Source: CAD feature listing. Evaluate the final solid. Frame: model axes, mm. A direction names the side the tool comes from. Round coordinates to 2 decimals unless told otherwise and drop trailing zeros. Loops run counter-clockwise (first coordinate to the right, second up) from the corner with the lowest first, then second, coordinate; pieces in that order, holes last. Notation, with made-up numbers: M -38.75,-36 L -33.75,-36 A3 cw -33.75,-32 Z; hole C 65.5,-8.75 d5. An arc over 180 degrees is marked long. Answer as a JSON object with one key per item and string values.
from build123d import *

# Parameters (mm, degrees)
SKETCH_1_R          = 30
SKETCH_1_R_2        = 1.5
SKETCH_1_R_3        = 3.5
EXTRUDE_1_DEPTH     = 20
SKETCH_2_R          = 21
CUT_EXTRUDE_1_DEPTH = 17
CUT_EXTRUDE_START   = -0.1
SKETCH_3_R          = 30
SKETCH_3_R_2        = 22.5
CUT_EXTRUDE_2_DEPTH = 0.1
FILLET_1_R          = 0.5


with BuildPart() as part:
    # 草图1 → 凸台-拉伸1 (new body)
    with BuildSketch(Plane(origin=(0, 0, 0), x_dir=(1, 0, 0), z_dir=(0, 1, 0))):
        with Locations(Location((0, 0, 0), (0, 0, 270))):
            Circle(SKETCH_1_R)
        with Locations(Location((0, 6, 0), (0, 0, 270))):
            Circle(SKETCH_1_R_2, mode=Mode.SUBTRACT)
        with Locations(Location((0, 0, 0), (0, 0, 270))):
            Circle(SKETCH_1_R_3, mode=Mode.SUBTRACT)
        with Locations(Location((6, 0, 0), (0, 0, 270))):
            Circle(SKETCH_1_R_2, mode=Mode.SUBTRACT)
        with Locations(Location((0, -6, 0), (0, 0, 270))):
            Circle(SKETCH_1_R_2, mode=Mode.SUBTRACT)
        with Locations(Location((-6, 0, 0), (0, 0, 270))):
            Circle(SKETCH_1_R_2, mode=Mode.SUBTRACT)
    extrude(amount=EXTRUDE_1_DEPTH)

    # 草图2 → 切除-拉伸1 (cut)
    with BuildSketch(Plane(origin=(0, 0, 0), x_dir=(-1, 0, 0), z_dir=(0, -1, 0))):
        with Locations(Location((0, 0, 0), (0, 0, 90))):
            Circle(SKETCH_2_R)
    extrude(amount=-CUT_EXTRUDE_1_DEPTH, mode=Mode.SUBTRACT)

    # 草图3 → 切除-拉伸2 (cut)
    with BuildSketch(Plane(origin=(0, 20, 0), x_dir=(1, 0, 0), z_dir=(0, 1, 0)).offset(CUT_EXTRUDE_START)):
        with Locations(Location((0, 0, 0), (0, 0, 270))):
            Circle(SKETCH_3_R)
        with Locations(Location((0, 0, 0), (0, 0, 270))):
            Circle(SKETCH_3_R_2, mode=Mode.SUBTRACT)
    extrude(amount=CUT_EXTRUDE_2_DEPTH, mode=Mode.SUBTRACT)

    # 圆角1
    fillet_1_edges = [part.edges().sort_by_distance(p)[0] for p in [
        (0, 0, -30),
        (0, 19.9, -30),
    ]]
    fillet(fillet_1_edges, radius=FILLET_1_R)


solid = part.part
Item 1: Pull-direction query (Z, two-part tool) for faces 4 (the flat face through (0, 17, -4)), 5 (the cylindrical face through (1.32, 9.82, -29.97)), 6 (the cylindrical face through (-3.417, 18.479, -0.759)), 7 (the flat face through (20, 0, -7)); classes: pulls with the +Z half, pulls with the -Z half, needs draft (parallel to the pull), parting line crosses it, or undercut.
Answer sheet:
{"face 4": "undercut", "face 5": "parting line crosses it", "face 6": "undercut", "face 7": "needs draft"}
Item 2: Contact query for flat-ended pins moving along their axis: pin 1 Ø2 at (x, y) = (13.5, 15.5) entering from +Z; pin 2 Ø1.5 at (y, z) = (11.5, 18.5) entering from -X; pin 3 Ø6 at (y, z) = (10.5, 5) entering from +X. Output: stop coordinate, or through.
Answer sheet:
{"pin 1": "stops at z = 27.27", "pin 2": "stops at x = -24.19", "pin 3": "stops at x = 29.93"}
Item 3: Section A-A on z = 0. Return the cut outline in (x, y).
Answer sheet:
{"outline": "M -30,0.5 A0.5 ccw -29.5,0 L -21,0 L -21,17 L -7.5,17 L -7.5,20 L -22.5,20 L -22.5,19.9 L -29.5,19.9 A0.5 ccw -30,19.4 Z; M -4.5,17 L -3.5,17 L -3.5,20 L -4.5,20 Z; M 3.5,17 L 4.5,17 L 4.5,20 L 3.5,20 Z; M 7.5,17 L 21,17 L 21,0 L 29.5,0 A0.5 ccw 30,0.5 L 30,19.4 A0.5 ccw 29.5,19.9 L 22.5,19.9 L 22.5,20 L 7.5,20 Z"}
Item 4: Section B-B on y = 9.5. Return the cut outline in (x, z).
Answer sheet:
{"outline": "C 0,0 d60; hole C 0,0 d42"}
Item 5: Line query: probe 1 along X at (y, z) = (18.7, 0); probe 2 along X at (y, z) = (7.75, 0.5); probe 3 along Y at (x, z) = (-25.5, -6). Output: solid intervals per line, ascending. Write a range as from..to.
Answer sheet:
{"probe 1": "x = -30..-7.5, -4.5..-3.5, 3.5..4.5, 7.5..30", "probe 2": "x = -30..-20.99, 20.99..30", "probe 3": "y = 0..19.9"}
Item 6: Access query for faces 1 (the cylindrical face through (6.31, 8.38, -20.03)), 2 (the flat face through (-22, 19.9, -7)), 3 (the flat face through (-5, 20, 5)). Directions: +Z, -Z, +X, -X, +Y, -Y. A direction counts if a zero-diameter tool reaches every point of the face in a straight line with its end or side. Return the directions, or none.
Answer sheet:
{"face 1": "-Y", "face 2": "+Y", "face 3": "+Z, -Z, +X, -X, +Y"}
